Verification items for the finished model (mm, model axes). A direction names the side the tool comes from. Round coordinates to 2 decimals unless told otherwise and drop trailing zeros. Write each loop counter-clockwise with the first axis right and the second up, starting at its lowest first coordinate (ties: lowest second). Pieces come first, ordered by that corner, then holes. Notation, with made-up numbers: (41.25, 40) - (86.25, 40) arc R13 ccw to (86.25, 61) - close; hole circle Ø3 at (32, 32.5). An arc over 180 degrees is marked (long way). Answer as a JSON object with one key per item and string values. Group by question number.
1) Set-up check for faces 1 (the flat face through (-9, 6, 40)), 2 (the flat face through (-9, -6, 190)), 3 (the flat face through (3, -10, 40)), 4 (the flat face through (-9, -6, 40)): record each of +Z, -Z, +X, -X, +Y, -Y from which the full face is reachable in a straight line by a thin tool's end or side.
2) Thickness scan on line 1 (X direction, y = -8, z = 127); line 2 (Y direction, x = -0.5, z = 60.5); line 3 (Z direction, x = -9.5, y = -6.75). Record the ranges inside material, lowest first.
3) Section check A-A (y = 0). Enter the section's corners in (x, z), then the cut area to 3 significant figures.
4) Section check B-B (z = 95.5). Enter the section's corners in (x, y), then the cut area to 4 significant figures.
5) Go/stop test with flat-tipped pins: pin 1 Ø10 at (x, y) = (6, 1) entering from -Z; pin 2 Ø1 at (x, y) = (4.5, 10.5) entering from -Z; pin 3 Ø1.1 at (x, y) = (10.5, 0.5) entering from +Z; pin 4 Ø1.1 at (x, z) = (11.5, 142) entering from +Y. Record where each tip stops, or that it passes through.
```python
from build123d import *

# Parameters (mm, degrees)
SKETCH1_R           = 10
BOSS_EXTRUDE1_DEPTH = 40
BOSS_EXTRUDE2_START = 40
SKETCH1_3_R         = 10
SKETCH1_3_W         = 4
SKETCH1_3_H         = 4
BOSS_EXTRUDE2_DEPTH = 150
BOSS_EXTRUDE3_START = 190
SKETCH1_4_R         = 10
BOSS_EXTRUDE3_DEPTH = 25
CHAMFER1_SIZE       = 1


with BuildPart() as part:
    # Sketch1 → Boss-Extrude1 (new body)
    with BuildSketch(Plane.XY):
        Circle(SKETCH1_R)
    extrude(amount=BOSS_EXTRUDE1_DEPTH)

    # Sketch1_3 → Boss-Extrude2 (add)
    with BuildSketch(Plane.XY.offset(BOSS_EXTRUDE2_START)):
        Circle(SKETCH1_3_R)
        Polygon((4.374248988, -6.990418142), (0.570022922, -8.226486119), (1.8060909, -12.030712184), (5.610316965, -10.794644207), align=None)
        with Locations((10, 0)):
            Rectangle(SKETCH1_3_W, SKETCH1_3_H)
        Polygon((-5.29656545, -6.320316007), (-7.64770646, -3.08424803), (-10.883774437, -5.435389039), (-8.532633428, -8.671457016), align=None)
        Polygon((-7.64770646, 3.08424803), (-5.29656545, 6.320316007), (-8.532633428, 8.671457016), (-10.883774437, 5.435389039), align=None)
        Polygon((0.570022922, 8.226486119), (4.374248988, 6.990418142), (5.610316965, 10.794644207), (1.8060909, 12.030712184), align=None)
    extrude(amount=BOSS_EXTRUDE2_DEPTH)

    # Sketch1_4 → Boss-Extrude3 (add)
    with BuildSketch(Plane.XY.offset(BOSS_EXTRUDE3_START)):
        Circle(SKETCH1_4_R)
    extrude(amount=BOSS_EXTRUDE3_DEPTH)

    # Chamfer1
    chamfer1_edges = [part.edges().sort_by_distance(p)[0] for p in [
        (-10, 0, 0),
        (-10, 0, 215),
    ]]
    chamfer(chamfer1_edges, length=CHAMFER1_SIZE)


solid = part.part
```
Returned:
{
 "1": {"face 1": "-Z, -X, +Y", "face 2": "+Z, -X, -Y", "face 3": "-Z, +X, -Y", "face 4": "-Z, -X, -Y"},
 "2": {"line 1": "-9.02 to -7.61, -6 to 6", "line 2": "-9.99 to 9.99", "line 3": "40 to 190"},
 "3": {"outline": "(-10, 1) - (-9, 0) - (9, 0) - (10, 1) - (10, 40) - (12, 40) - (12, 190) - (10, 190) - (10, 214) - (9, 215) - (-9, 215) - (-10, 214) - close", "area": "4,600 mm2"},
 "4": {"outline": "(-10.88, -5.44) - (-8.53, -8.67) - (-6.75, -7.38) arc R10 ccw to (1.13, -9.94) - (1.81, -12.03) - (5.61, -10.79) - (4.93, -8.7) arc R10 ccw to (9.8, -2) - (12, -2) - (12, 2) - (9.8, 2) arc R10 ccw to (4.93, 8.7) - (5.61, 10.79) - (1.81, 12.03) - (1.13, 9.94) arc R10 ccw to (-6.75, 7.38) - (-8.53, 8.67) - (-10.88, 5.44) - (-9.1, 4.14) arc R10 ccw to (-9.1, -4.14) - close", "area": "355.5 mm2"},
 "5": {"pin 1": "z = 0", "pin 2": "z = 40", "pin 3": "z = 214.04", "pin 4": "y = 2"}
}
